Design review of the part built by this model. Coordinates are the model's own, in mm. Face numbers are marked on the shaded views. A direction names the side the tool comes from. Round coordinates to 2 decimals unless told otherwise and drop trailing zeros. Write each loop counter-clockwise with the first axis right and the second up, starting at its lowest first coordinate (ties: lowest second). Pieces come first, ordered by that corner, then holes. Notation, with made-up numbers: (89, 66.25) -> (102, 66.25) arc R32 cw to (102, 101.25) -> close; hole circle Ø2 at (88.5, 36). An arc over 180 degrees is marked (long way). One line per question, with ' | ' between items. Start each with the question number.
1) Consider section C-C (x = 6). Give the boundary of the cut face in (y, z).
2) Consider section B-B (y = 36.1). Count the separate pieces of the cut face and the enclosed holes in it, then the cut area to 3 significant figures.
3) Mouldability with a two-part tool opening along X and no side actions: class the marked faces 1, 2 and 3 as +X half, -X half, draft (parallel to the pull), parting line (faces both ways), or undercut.
4) Consider section D-D (x = 24.5). Give the boundary of the cut face in (y, z), then the cut area to 3 significant figures.
5) For the marked faces 4, 5 and 6, list the 3-axis set-ups (+Z, -Z, +X, -X, +Y, -Y) from which the entire face can be reached by the end or side of a thin tool; tool diameter is ignored.
6) Insertion check: pin 1 Ø12.5 at (y, z) = (36.1, 26.04) entering from +X; pin 2 Ø12 at (y, z) = (-7.5, -9) entering from +X; pin 3 Ø5 at (x, z) = (2.5, -22) entering from +Y; pin 4 Ø12 at (x, z) = (17, 7) entering from +Y. Each pin has a flat end and moves straight along its axis. Give the tip position at first contact, or say it passes through.
7) For probe 1 along Z at (x, y) = (2, 30); probe 2 along Z at (x, y) = (26, 36.1); probe 3 along Z at (x, y) = (19, 36), list the stretches that pass through material, from the lowest coordinate up.
8) Consider section A-A (y = 21). Give the boundary of the cut face in (x, z), then the cut area to 3 significant figures.
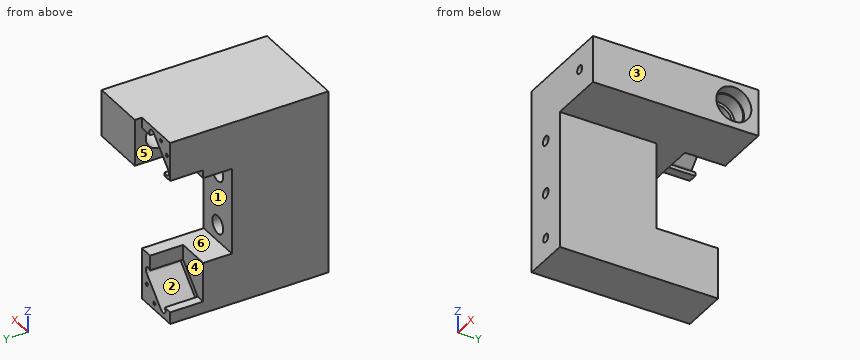
```python
from build123d import *

# Parameters (mm, degrees)
BOSS_EXTRUDE1_DEPTH            = 45
SKETCH2_W                      = 17
SKETCH2_H                      = 31.401973819
CUT_EXTRUDE1_DEPTH             = 25
BOSS_EXTRUDE2_DEPTH            = 15
SKETCH5_W                      = 17
SKETCH5_H                      = 18.598026181
CUT_EXTRUDE2_DEPTH             = 2.6
CUT_EXTRUDE3_DEPTH             = 12
CUT_EXTRUDE4_DEPTH             = 14.6
SKETCH4_R                      = 6.35
CUT_EXTRUDE6_DEPTH             = 4.4
SKETCH11_R                     = 6
CUT_EXTRUDE7_DEPTH             = 5
SM05_TAPPED_HOLE1_D            = 12.7
SM05_TAPPED_HOLE1_DEPTH        = 3
SM05_TAPPED_HOLE1_TIP          = 3.815464931
CUT_EXTRUDE9_DEPTH             = 12.5
CUT_EXTRUDE10_DEPTH            = 0.5
CUT_EXTRUDE11_DEPTH            = 2.6
SKETCH18_R                     = 4.89982915
CUT_EXTRUDE12_DEPTH            = 10.6
CBORE_FOR_M3_SHCS1_D           = 3.4
CBORE_FOR_M3_SHCS1_DEPTH       = 35
CBORE_FOR_M3_SHCS1_CBORE_D     = 6.5
CBORE_FOR_M3_SHCS1_CBORE_DEPTH = 25
F_3_0MM_DOWEL_HOLE1_D          = 3
F_3_0MM_DOWEL_HOLE1_DEPTH      = 5.2
F_3_0MM_DOWEL_HOLE1_TIP        = 0.901290929
M1_6_TAPPED_HOLE1_D            = 1.25
M1_6_TAPPED_HOLE1_DEPTH        = 4.25
M1_6_TAPPED_HOLE1_TIP          = 0.375537887
M1_6_TAPPED_HOLE2_D            = 1.25
M1_6_TAPPED_HOLE2_DEPTH        = 4.25
M1_6_TAPPED_HOLE2_TIP          = 0.375537887


with BuildPart() as part:
    # Sketch1 → Boss-Extrude1 (new body)
    with BuildSketch(Plane(origin=(0, 0, 0), x_dir=(1, 0, 0), z_dir=(0, 1, 0))):
        Polygon((27.364828995, -34.317342946), (-9.635171005, -34.317342946), (-9.635171005, 32.682657054), (7.364828995, 32.682657054), (7.364828995, -17.317342946), (27.364828995, -17.317342946), align=None)
    extrude(amount=BOSS_EXTRUDE1_DEPTH)

    # Sketch2 → Cut-Extrude1 (cut)
    with BuildSketch(Plane(origin=(0, 45, 0), x_dir=(1, 0, 0), z_dir=(0, 1, 0))):
        with Locations((-1.135171005, -1.616356037)):
            Rectangle(SKETCH2_W, SKETCH2_H)
    extrude(amount=-CUT_EXTRUDE1_DEPTH, mode=Mode.SUBTRACT)

    # Sketch3 → Boss-Extrude2 (add)
    with BuildSketch(Plane.XZ):
        Polygon((27.364828995, 34.317342946), (-9.635171005, 34.317342946), (-9.635171005, -32.682657054), (7.364828995, -32.682657054), (7.364828995, 17.317342946), (27.364828995, 17.317342946), align=None)
    extrude(amount=BOSS_EXTRUDE2_DEPTH)

    # Sketch5 → Cut-Extrude2 (cut)
    with BuildSketch(Plane(origin=(0, 45, 0), x_dir=(1, 0, 0), z_dir=(0, 1, 0))):
        with Locations((-1.135171005, 23.383643964)):
            Rectangle(SKETCH5_W, SKETCH5_H)
    extrude(amount=-CUT_EXTRUDE2_DEPTH, mode=Mode.SUBTRACT)

    # Sketch6 → Cut-Extrude3 (cut)
    with BuildSketch(Plane(origin=(0, 42.4, 0), x_dir=(1, 0, 0), z_dir=(0, 1, 0))):
        Polygon((-9.635171005, 28.375993351), (-9.635171005, 14.084630873), (2.47645738, 14.084630873), (2.47645738, 19.537158586), (-6.362377384, 28.375993351), align=None)
    extrude(amount=-CUT_EXTRUDE3_DEPTH, mode=Mode.SUBTRACT)

    # Sketch7 → Cut-Extrude4 (cut)
    with BuildSketch(Plane(origin=(0, 45, 0), x_dir=(1, 0, 0), z_dir=(0, 1, 0))):
        with BuildLine():
            Line((2.47645738, -30.462841414), (7.364828995, -30.462841414))
            Line((7.364828995, -30.462841414), (7.364828995, -17.317342946))
            Line((7.364828995, -17.317342946), (-9.635171005, -17.317342946))
            Line((-9.635171005, -17.317342946), (-9.635171005, -20.274833742))
            Line((-9.635171005, -20.274833742), (-6.362377384, -20.274833742))
            Line((-6.362377384, -20.274833742), (-6.362377384, -21.624006649))
            ThreePointArc((-6.362377384, -21.624006649), (-8.483697728, -21.624006649), (-8.483697728, -23.745326993))
            Line((-8.483697728, -23.745326993), (0.355137037, -32.584161758))
            ThreePointArc((0.355137037, -32.584161758), (2.47645738, -32.584161758), (2.47645738, -30.462841414))
        make_face()
    extrude(amount=-CUT_EXTRUDE4_DEPTH, mode=Mode.SUBTRACT)

    # Sketch4 → Cut-Extrude6 (cut)
    with BuildSketch(Plane(origin=(27.364828995, 0, 0), x_dir=(0, 0, -1), z_dir=(1, 0, 0))):
        with Locations((-26.043424032, 36.1)):
            Circle(SKETCH4_R)
    extrude(amount=-CUT_EXTRUDE6_DEPTH, mode=Mode.SUBTRACT)

    # Sketch11 → Cut-Extrude7 (cut)
    with BuildSketch(Plane(origin=(22.964828995, 0, 0), x_dir=(0, 0, -1), z_dir=(1, 0, 0))):
        with Locations((-26.043424032, 36.1)):
            Circle(SKETCH11_R)
    extrude(amount=-CUT_EXTRUDE7_DEPTH, mode=Mode.SUBTRACT)

    # SM05 Tapped Hole1
    with Locations(Plane(origin=(27.364828995, 0, 0), x_dir=(0, 0, -1), z_dir=(1, 0, 0))):
        with Locations((-26.043424032, 36.1)):
            Hole(SM05_TAPPED_HOLE1_D / 2, depth=SM05_TAPPED_HOLE1_DEPTH)
            with Locations((0, 0, -(SM05_TAPPED_HOLE1_DEPTH + SM05_TAPPED_HOLE1_TIP / 2))):  # 118° drill point
                Cone(0, SM05_TAPPED_HOLE1_D / 2, SM05_TAPPED_HOLE1_TIP, mode=Mode.SUBTRACT)

    # Sketch15 → Cut-Extrude9 (cut)
    with BuildSketch(Plane(origin=(0, 42.4, 0), x_dir=(1, 0, 0), z_dir=(0, 1, 0))):
        with BuildLine():
            Line((-4.241057041, 30.497313694), (4.597777724, 21.658478929))
            ThreePointArc((4.597777724, 21.658478929), (4.597777724, 19.537158586), (2.47645738, 19.537158586))
            Line((2.47645738, 19.537158586), (-6.362377384, 28.375993351))
            ThreePointArc((-6.362377384, 28.375993351), (-6.362377384, 30.497313694), (-4.241057041, 30.497313694))
        make_face()
    extrude(amount=-CUT_EXTRUDE9_DEPTH, mode=Mode.SUBTRACT)

    # Sketch16 → Cut-Extrude10 (cut)
    with BuildSketch(Plane(origin=(0, 30.4, 0), x_dir=(1, 0, 0), z_dir=(0, 1, 0))):
        with BuildLine():
            Line((-6.362377384, -21.624006649), (2.47645738, -30.462841414))
            ThreePointArc((2.47645738, -30.462841414), (2.47645738, -32.584161758), (0.355137037, -32.584161758))
            Line((0.355137037, -32.584161758), (-8.483697728, -23.745326993))
            ThreePointArc((-8.483697728, -23.745326993), (-8.483697728, -21.624006649), (-6.362377384, -21.624006649))
        make_face()
    extrude(amount=-CUT_EXTRUDE10_DEPTH, mode=Mode.SUBTRACT)

    # Sketch17 → Cut-Extrude11 (cut)
    with BuildSketch(Plane(origin=(0, 45, 0), x_dir=(1, 0, 0), z_dir=(0, 1, 0))):
        with BuildLine():
            Line((7.364828995, -30.462841414), (7.364828995, -34.317342946))
            Line((7.364828995, -34.317342946), (-9.635171005, -34.317342946))
            Line((-9.635171005, -34.317342946), (-9.635171005, -20.274833742))
            Line((-9.635171005, -20.274833742), (-6.362377384, -20.274833742))
            Line((-6.362377384, -20.274833742), (-6.362377384, -21.624006649))
            ThreePointArc((-6.362377384, -21.624006649), (-8.483697728, -21.624006649), (-8.483697728, -23.745326993))
            Line((-8.483697728, -23.745326993), (0.355137037, -32.584161758))
            ThreePointArc((0.355137037, -32.584161758), (2.47645738, -32.584161758), (2.47645738, -30.462841414))
            Line((2.47645738, -30.462841414), (7.364828995, -30.462841414))
        make_face()
    extrude(amount=-CUT_EXTRUDE11_DEPTH, mode=Mode.SUBTRACT)

    # Sketch18 → Cut-Extrude12 (cut)
    with BuildSketch(Plane(origin=(17.964828995, 0, 0), x_dir=(0, 0, -1), z_dir=(1, 0, 0))):
        with Locations((-26.043424032, 36.1)):
            Circle(SKETCH18_R)
    extrude(amount=-CUT_EXTRUDE12_DEPTH, mode=Mode.SUBTRACT)

    # CBORE for M3 SHCS1
    with Locations(Plane(origin=(0, 20, 0), x_dir=(1, 0, 0), z_dir=(0, 1, 0))):
        with Locations((-1.135171005, 8.084630873), (-1.135171005, -11.317342946)):
            CounterBoreHole(CBORE_FOR_M3_SHCS1_D / 2, CBORE_FOR_M3_SHCS1_CBORE_D / 2, CBORE_FOR_M3_SHCS1_CBORE_DEPTH, depth=CBORE_FOR_M3_SHCS1_DEPTH)

    # Ø3.0mm Dowel Hole1
    with Locations(Plane(origin=(0, -15, 0), x_dir=(-1, 0, 0), z_dir=(0, -1, 0))):
        with Locations((-19.364828995, -26.317342946), (1.135171005, 24.682657054)):
            Hole(F_3_0MM_DOWEL_HOLE1_D / 2, depth=F_3_0MM_DOWEL_HOLE1_DEPTH)
            with Locations((0, 0, -(F_3_0MM_DOWEL_HOLE1_DEPTH + F_3_0MM_DOWEL_HOLE1_TIP / 2))):  # 118° drill point
                Cone(0, F_3_0MM_DOWEL_HOLE1_D / 2, F_3_0MM_DOWEL_HOLE1_TIP, mode=Mode.SUBTRACT)

    # M1.6 Tapped Hole1
    with Locations(Plane(origin=(0, 42.4, 0), x_dir=(1, 0, 0), z_dir=(0, 1, 0))):
        with Locations((-0.132659145, 30.363070903), (4.463534932, 25.766876825)):
            Hole(M1_6_TAPPED_HOLE1_D / 2, depth=M1_6_TAPPED_HOLE1_DEPTH)
            with Locations((0, 0, -(M1_6_TAPPED_HOLE1_DEPTH + M1_6_TAPPED_HOLE1_TIP / 2))):  # 118° drill point
                Cone(0, M1_6_TAPPED_HOLE1_D / 2, M1_6_TAPPED_HOLE1_TIP, mode=Mode.SUBTRACT)

    # M1.6 Tapped Hole2
    with Locations(Plane(origin=(0, 42.4, 0), x_dir=(1, 0, 0), z_dir=(0, 1, 0))):
        with Locations((-4.135171005, -32.107144182), (-7.635171005, -28.607144182)):
            Hole(M1_6_TAPPED_HOLE2_D / 2, depth=M1_6_TAPPED_HOLE2_DEPTH)
            with Locations((0, 0, -(M1_6_TAPPED_HOLE2_DEPTH + M1_6_TAPPED_HOLE2_TIP / 2))):  # 118° drill point
                Cone(0, M1_6_TAPPED_HOLE2_D / 2, M1_6_TAPPED_HOLE2_TIP, mode=Mode.SUBTRACT)


solid = part.part
```
From the geometry:
1) outline: (-15, -32.68) -> (42.4, -32.68) -> (42.4, -14.08) -> (20, -14.08) -> (20, 17.32) -> (30.4, 17.32) -> (30.4, 30.46) -> (42.4, 30.46) -> (42.4, 34.32) -> (-15, 34.32) -> close
2) separate pieces: 3 | enclosed holes: 0 | area: 351 mm2
3) face 1: draft | face 2: undercut | face 3: +X half
4) outline: (-15, 17.32) -> (45, 17.32) -> (45, 34.32) -> (-15, 34.32) -> close; hole circle Ø12.7 at (36.1, 26.04) | area: 893 mm2
5) face 4: -X, +Y | face 5: +Y | face 6: +X, -X, +Y
6) pin 1: stops at x = 22.96 | pin 2: stops at x = 7.36 | pin 3: stops at y = 42.4 | pin 4: passes through
7) probe 1: z = -32.68 to -24.26, -20.01 to -14.08, 17.32 to 29.99, 32.91 to 34.32 | probe 2: z = 17.32 to 19.69, 32.39 to 34.32 | probe 3: z = 17.32 to 20.04, 32.04 to 34.32
8) outline: (-9.64, -32.68) -> (7.36, -32.68) -> (7.36, -14.08) -> (-9.64, -14.08) -> close; (-9.64, 17.32) -> (27.36, 17.32) -> (27.36, 34.32) -> (-9.64, 34.32) -> close | area: 945 mm2
